Input: part model. Units: mm. Frame: model coordinates. A direction names the side the tool comes from. Coordinates: 2 decimals unless noted, no trailing zeros. Loops run counter-clockwise (first coordinate to the right, second up) from the corner with the lowest first, then second, coordinate; pieces in that order, holes last.
```python
from build123d import *

# Parameters (mm, degrees)
SCHIZZO1_W                   = 67
SCHIZZO1_H                   = 130
ESTRUSIONE_ESTRUSIONE1_DEPTH = 1
RACCORDO1_R                  = 1
RACCORDO2_R                  = 1
TAGLIO_ESTRUSIONE1_REACH     = 75.132
SCHIZZO2_W                   = 6
SCHIZZO2_H                   = 52
SCHIZZO3_W                   = 7.019243903
SCHIZZO3_H                   = 58.993368718
SCHIZZO3_W_2                 = 11.981035511
SCHIZZO3_H_2                 = 5
ESTRUSIONE_ESTRUSIONE2_DEPTH = 14.5
TAGLIO_ESTRUSIONE3_REACH     = 76.75
SCHIZZO8_W                   = 3.086111391
SCHIZZO8_H                   = 8.391810393
TAGLIO_ESTRUSIONE4_REACH     = 76.75
SCHIZZO10_W                  = 7.563253313
SCHIZZO10_H                  = 2.803619763
SCHIZZO11_R                  = 0.5
TAGLIO_ESTRUSIONE5_DEPTH     = 10
SCHIZZO12_R                  = 0.5
TAGLIO_ESTRUSIONE6_DEPTH     = 10
SCHIZZO13_R                  = 0.5
TAGLIO_ESTRUSIONE7_DEPTH     = 10
SCHIZZO14_R                  = 0.5
TAGLIO_ESTRUSIONE8_DEPTH     = 10


# Some blends are built 0.0001 mm under size
with BuildPart() as part:
    # Schizzo1 → Estrusione-Estrusione1 (new body)
    with BuildSketch(Plane.XY):
        Rectangle(SCHIZZO1_W, SCHIZZO1_H)
    extrude(amount=ESTRUSIONE_ESTRUSIONE1_DEPTH)

    # Raccordo1
    raccordo1_edges = [part.edges().sort_by_distance(p)[0] for p in [
        (0, 65, 1),
        (33.5, 0, 1),
        (0, -65, 1),
        (-33.5, 0, 1),
    ]]
    fillet(raccordo1_edges, radius=RACCORDO1_R - 0.0001)  # a hair under: the kernel refuses the full size

    # Raccordo2
    # the kernel refuses this fillet: 1 mm, written as the material it takes off along each edge
    with BuildSketch(Plane(origin=(32.5, -64, 1), x_dir=(0, -1, 0), z_dir=(-1, 0, 0))) as raccordo2_piece_1:
        with BuildLine():
            CenterArc((0.0001, -0.9999), 0.9999, 0, 90)
            Line((1, -0.9999), (1, 0))
            Line((1, 0), (0.0001, 0))
        make_face()
    revolve(axis=Axis((32.5, -64, 1), (0, 0, 1)), revolution_arc=90, mode=Mode.SUBTRACT)
    with BuildSketch(Plane(origin=(-32.5, -64, 1), x_dir=(-1, 0, 0), z_dir=(0, 1, 0))) as raccordo2_piece_2:
        with BuildLine():
            CenterArc((0.0001, -0.9999), 0.9999, 0, 90)
            Line((1, -0.9999), (1, 0))
            Line((1, 0), (0.0001, 0))
        make_face()
    revolve(axis=Axis((-32.5, -64, 1), (0, 0, 1)), revolution_arc=90, mode=Mode.SUBTRACT)
    with BuildSketch(Plane(origin=(32.5, 64, 1), x_dir=(1, 0, 0), z_dir=(0, -1, 0))) as raccordo2_piece_3:
        with BuildLine():
            CenterArc((0.0001, -0.9999), 0.9999, 0, 90)
            Line((1, -0.9999), (1, 0))
            Line((1, 0), (0.0001, 0))
        make_face()
    revolve(axis=Axis((32.5, 64, 1), (0, 0, 1)), revolution_arc=90, mode=Mode.SUBTRACT)
    with BuildSketch(Plane(origin=(-32.5, 64, 1), x_dir=(0, 1, 0), z_dir=(1, 0, 0))) as raccordo2_piece_4:
        with BuildLine():
            CenterArc((0.0001, -0.9999), 0.9999, 0, 90)
            Line((1, -0.9999), (1, 0))
            Line((1, 0), (0.0001, 0))
        make_face()
    revolve(axis=Axis((-32.5, 64, 1), (0, 0, 1)), revolution_arc=90, mode=Mode.SUBTRACT)
    with BuildSketch(Plane(origin=(-33.5, 65, -2.5), x_dir=(1, 0, 0), z_dir=(0, 0, 1)), Plane(origin=(-33.5, -65, -2.5), x_dir=(0, 1, 0), z_dir=(0, 0, 1))) as raccordo2_piece_5:
        with BuildLine():
            CenterArc((RACCORDO2_R, -RACCORDO2_R), RACCORDO2_R, 90, 90)
            Line((0, -RACCORDO2_R), (0, 0))
            Line((0, 0), (RACCORDO2_R, 0))
        make_face()
    extrude(amount=3.5, mode=Mode.SUBTRACT)
    with BuildSketch(Plane(origin=(33.5, 65, -2.5), x_dir=(-1, 0, 0), z_dir=(0, 0, 1)), Plane(origin=(33.5, -65, -2.5), x_dir=(0, 1, 0), z_dir=(0, 0, 1))) as raccordo2_piece_6:
        with BuildLine():
            CenterArc((RACCORDO2_R, RACCORDO2_R), RACCORDO2_R, 180, 90)
            Line((0, RACCORDO2_R), (0, 0))
            Line((0, 0), (RACCORDO2_R, 0))
        make_face()
    extrude(amount=3.5, mode=Mode.SUBTRACT)

    # Schizzo2 → Taglio-Estrusione1 (cut, up to next)
    with BuildSketch(Plane.XY.offset(1), mode=Mode.PRIVATE) as taglio_estrusione1_sk1:
        with Locations((7.5, -29)):
            Rectangle(SCHIZZO2_W, SCHIZZO2_H)
    taglio_estrusione1_tool1 = extrude(taglio_estrusione1_sk1.sketch, amount=-TAGLIO_ESTRUSIONE1_REACH, mode=Mode.PRIVATE) & part.part
    add(taglio_estrusione1_tool1.solids().sort_by_distance((7.5, -29, 1))[0], mode=Mode.SUBTRACT)

    # Schizzo3 → Estrusione-Estrusione2 (add)
    with BuildSketch(Plane(origin=(0, 0, 0), x_dir=(-1, 0, 0), z_dir=(0, 0, -1))):
        Polygon((-32.5, -64), (-10.5, -64), (-10.5, 5.006631282), (-4.308376316, 5.006631282), (-4.308376316, 9.963903227), (-32.5, 9.963903227), (-32.5, 5), align=None)
        with Locations((28.990378048, 34.503315641)):
            Rectangle(SCHIZZO3_W, SCHIZZO3_H)
        with Locations((-3.813832367, 61.5)):
            Rectangle(SCHIZZO3_W_2, SCHIZZO3_H_2)
    extrude(amount=ESTRUSIONE_ESTRUSIONE2_DEPTH)

    # Schizzo8 → Taglio-Estrusione3 (cut, up to next)
    with BuildSketch(Plane.XY.offset(1), mode=Mode.PRIVATE) as taglio_estrusione3_sk1:
        with Locations((-17.456944304, -35.054094803)):
            Rectangle(SCHIZZO8_W, SCHIZZO8_H)
    taglio_estrusione3_tool1 = extrude(taglio_estrusione3_sk1.sketch, amount=-TAGLIO_ESTRUSIONE3_REACH, mode=Mode.PRIVATE) & part.part
    add(taglio_estrusione3_tool1.solids().sort_by_distance((-17.456944, -35.054095, 1))[0], mode=Mode.SUBTRACT)

    # Schizzo10 → Taglio-Estrusione4 (cut, up to next)
    with BuildSketch(Plane.XY.offset(1), mode=Mode.PRIVATE) as taglio_estrusione4_sk1:
        with Locations((-22.018373344, -60.998190119)):
            Rectangle(SCHIZZO10_W, SCHIZZO10_H)
    taglio_estrusione4_tool1 = extrude(taglio_estrusione4_sk1.sketch, amount=-TAGLIO_ESTRUSIONE4_REACH, mode=Mode.PRIVATE) & part.part
    add(taglio_estrusione4_tool1.solids().sort_by_distance((-22.018373, -60.99819, 1))[0], mode=Mode.SUBTRACT)

    # Schizzo11 → Taglio-Estrusione5 (cut)
    with BuildSketch(Plane(origin=(32.5, 0, 0), x_dir=(0, 0, -1), z_dir=(1, 0, 0))):
        with Locations(Location((9, -26, 0), (0, 0, 90))):
            Circle(SCHIZZO11_R)
    extrude(amount=-TAGLIO_ESTRUSIONE5_DEPTH, mode=Mode.SUBTRACT)

    # Schizzo12 → Taglio-Estrusione6 (cut)
    with BuildSketch(Plane(origin=(0, 64, 0), x_dir=(1, 0, 0), z_dir=(0, 1, 0))):
        with Locations(Location((3.813832367, 9, 0), (0, 0, 270))):
            Circle(SCHIZZO12_R)
    extrude(amount=-TAGLIO_ESTRUSIONE6_DEPTH, mode=Mode.SUBTRACT)

    # Schizzo13 → Taglio-Estrusione7 (cut)
    with BuildSketch(Plane.ZY.offset(32.5)):
        with Locations((-9, 36)):
            Circle(SCHIZZO13_R)
    extrude(amount=-TAGLIO_ESTRUSIONE7_DEPTH, mode=Mode.SUBTRACT)

    # Schizzo14 → Taglio-Estrusione8 (cut)
    with BuildSketch(Plane.XZ.offset(64)):
        with Locations(Location((20.5, -9, 0), (0, 0, 270))):
            Circle(SCHIZZO14_R)
    extrude(amount=-TAGLIO_ESTRUSIONE8_DEPTH, mode=Mode.SUBTRACT)


solid = part.part
```
Item 1: Line query: L1, parallel to X at y = 61.95, z = -9; L2, parallel to Z at x = -28, y = 36; L3, parallel to X at y = -61, z = -9. Output: solid intervals per line, ascending.
Result:
L1: x = -32.5 to -25.48, -2.18 to 3.31, 4.31 to 9.8
L2: z = -14.5 to -9.5, -8.5 to 1
L3: x = 10.5 to 20, 21 to 32.5
Item 2: Mould query, pull axis X, two halves, no side actions, for faces 1 (the face through (9.804, 61, -7)), 2 (the face through (-2.177, 61, -7)), 3 (the face through (0, 1, 1)). Classes: +X half, -X half, draft (parallel to the pull), parting line (faces both ways), or undercut.
Result:
face 1: +X half
face 2: undercut
face 3: draft
Item 3: Section query B-B (z = -7.25). Output: boundary loops of the cut face in (x, y).
Result:
outline: (-32.5, 5.01) - (-25.48, 5.01) - (-25.48, 64) - (-32.5, 64) - close; (-2.18, 59) - (9.8, 59) - (9.8, 64) - (-2.18, 64) - close; (4.31, 5.01) - (10.5, 5.01) - (10.5, -64) - (32.5, -64) - (32.5, 9.96) - (4.31, 9.96) - close
Item 4: Contact query for flat-ended pins moving along their axis: P1, Ø2.5, axis at y = 8, z = -4, coming from the -X side; P2, Ø1.1, axis at x = -23.5, z = 0.5, coming from the +Y side; P3, Ø4, axis at x = -1, z = -11.5, coming from the -Y side; P4, Ø0.5, axis at x = -16.5, z = 0.5, coming from the -Y side. Output: stop coordinate, or through.
Result:
P1: stops at x = -32.5
P2: stops at y = 65
P3: stops at y = 59
P4: stops at y = -64.97
Item 5: Reachability of faces 4 (the face through (-32.5, 34, -7)), 5 (the face through (4.308, 7, -7)), 6 (the face through (22, -64, -7)), 7 (the face through (4, 59, -7)) from +Z, -Z, +X, -X, +Y, -Y: full face, straight path, thin tool, end or side. Return the list, or none.
Result:
face 4: -Z, -X, +Y, -Y
face 5: -Z, -Y
face 6: -Z, +X, -X, -Y
face 7: -Z, +X
